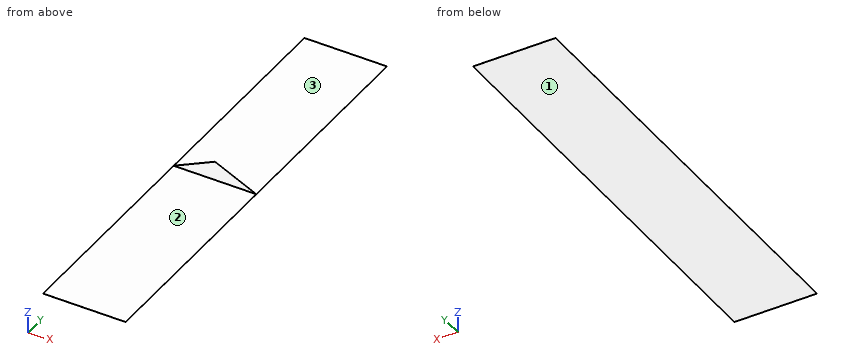
Autodesk Inventor part; units mm, degrees
ref_plane "YZ Plane" through (0, 0, 0) normal (1, 0, 0) x (0, 1, 0)
ref_plane "XZ Plane" through (0, 0, 0) normal (0, 1, 0) x (-1, 0, 0)
ref_plane "XY Plane" through (0, 0, 0) normal (0, 0, 1) x (1, 0, 0)
sketch "Sketch1" plane through (0, 0, 0) normal (0, 1, 0) x (-1, 0, 0)
  line L0 (7, 0) -> (-7, 0)
  arc A0 (-5, -3.7812) -> (5, -3.7812) centre (0, 9.3638) ccw
  line L1 (0, -4.7) -> (163.1354, -80.7713)
  line L2 (0, -4.7) -> (180, -4.7) construction
  line L3 (0, -4.7) -> (97.3734, -4.7) construction
  line L4 (0, -4.7) -> (-163.1354, -80.7713)
  line L5 (0, -4.7) -> (180, -4.7) construction
  line L6 (-163.1354, -80.7713) -> (163.1354, -80.7713)
  point P0 (0, 0)
extrude "Extrusion1" add sketch "Sketch1" along normal blind 0.1
sketch "Sketch3" plane through (163.1354, 0, -80.7713) normal (0, 0, -1) x (-1, 0, 0)
  line L0 (0, 0) -> (326.2708, 0)
  line L1 (326.2708, 0) -> (326.2708, 0.1)
  line L2 (0, 0.1) -> (326.2708, 0.1)
  line L3 (0, 0) -> (0, 0.1)
  point P0 (163.1354, 0)
extrude "Extrusion2" add sketch "Sketch3" along normal blind 0.1
sketch "Sketch4" plane through (163.1354, 0, -80.7713) normal (1, 0, 0) x (0, 0, -1)
  line L0 (-76.0713, 0) -> (0, 0)
  line L1 (-76.0713, 0) -> (0, -869.4988)
  line L2 (-76.0713, 0) -> (796.7488, 0) construction
  line L3 (-76.0713, 0) -> (0, 869.4988)
  line L4 (-76.0713, 0) -> (796.7488, 0) construction
  line L5 (0, 869.4988) -> (0, -869.4988)
  point P0 (-80.7713, 0)
  dimension "d10" = 85
  dimension "d11" = 85
extrude "Extrusion3" add sketch "Sketch4" along normal blind 0.1
sketch "Sketch5" plane through (163.1354, 0, -80.8713) normal (0, 0, -1) x (-1, 0, 0)
  line L0 (0, -869.4988) -> (0, 0)
  line L1 (0, 0.1) -> (0, 0)
  line L2 (0, 0.1) -> (0, 869.4988)
  line L3 (0, 0) -> (326.2708, 0)
  line L4 (0, -869.4988) -> (326.2708, -869.4988)
  line L5 (326.2708, -869.4988) -> (326.2708, 869.4988)
  line L6 (326.2708, 869.4988) -> (0, 869.4988)
  line L7 (0, 869.4988) -> (0, -869.4988)
  point P0 (163.1354, 0)
extrude "Extrusion4" add sketch "Sketch5" along normal blind 0.1
sketch "Sketch6" plane through (163.2354, 0, -80.7713) normal (1, 0, 0) x (0, 0, -1)
  line L0 (0, -869.4988) -> (0, 0)
  line L1 (-76.0713, 0) -> (0, -869.4988)
  line L2 (0, 869.4988) -> (-76.0713, 0)
  line L3 (0, 0.1) -> (0, 869.4988)
  line L4 (0, 0) -> (0, 0.1)
  point P0 (-80.7713, 0)
extrude "Extrusion5" cut sketch "Sketch6" against normal blind 0.1
properties part number "FOVcam"
Build history of the part. All positions in model axes, mm. Face numbers are marked on the shaded views. A direction names the side the tool comes from. Give positions to 0.01 mm unless a question says otherwise; leave off trailing zeros. Order: outer loops, then holes, each group sorted by start corner. A loop starts at its lowest first (then second) coordinate and runs counter-clockwise, first axis right, second up. Notation, with made-up numbers: M -5.75,-20 L 18.25,-20 A22 ccw 18.25,19 Z; hole C -6,35 d8. An arc over 180 degrees is marked long. Put each result on its own line as item: value.
Item 1: Slice it at B-B, the plane z = -56.5. Write the cut outline in (x, y).
From the geometry:
outline: M -111.09,0 L 111.09,0 L 111.09,0.1 L -111.09,0.1 Z
Item 2: 3-axis set-ups, long thin cutter, end or side, ignore diameter. For the marked faces 1, 2 and 3: which of +Z, -Z, +X, -X, +Y, -Y reach the whole face in a straight line?
From the geometry:
face 1: -Z, +X, -X, +Y, -Y
face 2: +Z, +X, -X, -Y
face 3: +Z, +X, -X, +Y
Item 3: Flat gauge pins, fed straight in: pin 1 Ø4 at (x, y) = (-102.5, 141.5) entering from +Z; pin 2 Ø10 at (x, z) = (24.5, -15) entering from +Y. Where does each tip first touch, or does it go through?
From the geometry:
pin 1: stops at z = -80.87
pin 2: stops at y = 0.1
Item 4: Slice it at C-C, the plane y = -465. Write the cut outline in (x, z), plus the area to 3 significant figures.
From the geometry:
outline: M -163.14,-80.97 L 163.14,-80.97 L 163.14,-80.87 L -163.14,-80.87 Z
area: 32.6 mm2
Item 5: Slice it at D-D, the plane x = 57.5. Write the cut outline in (y, z), plus the area to 3 significant figures.
From the geometry:
outline: M -869.5,-80.97 L 869.5,-80.97 L 869.5,-80.87 L 0.1,-80.87 L 0.1,-31.51 L 0,-31.51 L 0,-80.87 L -869.5,-80.87 Z
area: 179 mm2
Item 6: Slice it at A-A, the plane x = -19. Write the cut outline in (y, z), plus the area to 3 significant figures.
From the geometry:
outline: M -869.5,-80.97 L 869.5,-80.97 L 869.5,-80.87 L 0.1,-80.87 L 0.1,-13.56 L 0,-13.56 L 0,-80.87 L -869.5,-80.87 Z
area: 181 mm2
